from build123d import *

# Parameters (mm, degrees)
BOX_W             = 0.2
BOX_H             = 2.5
BOX_DEPTH         = 0.5
BOX001_W          = 2.5
BOX001_H          = 0.2
BOX001_DEPTH      = 0.5
CYLINDER_R        = 2.8
CYLINDER_DEPTH    = 1.65
CYLINDER001_R     = 1
CYLINDER001_DEPTH = 5
CHAMFER_SIZE      = 1.59
CHAMFER001_SIZE   = 0.1


with BuildPart() as obj1:
    # Box → Box (new body)
    with BuildSketch(Plane(origin=(-0.1, -1.25, 0), x_dir=(1, 0, 0), z_dir=(0, 0, 1))):
        with Locations((0.1, 1.25)):
            Rectangle(BOX_W, BOX_H)
    extrude(amount=BOX_DEPTH)


with BuildPart() as fusion:
    # Box001 → Box001 (new body)
    with BuildSketch(Plane(origin=(-1.25, -0.1, 0), x_dir=(1, 0, 0), z_dir=(0, 0, 1))):
        with Locations((1.25, 0.1)):
            Rectangle(BOX001_W, BOX001_H)
    extrude(amount=BOX001_DEPTH)

    # Fusion: union obj1
    add(obj1.part)


with BuildPart() as zylinder:
    # Cylinder → Cylinder (new body)
    with BuildSketch(Plane.XY):
        Circle(CYLINDER_R)
    extrude(amount=CYLINDER_DEPTH)


with BuildPart() as screw:
    # Cylinder001 → Cylinder001 (new body)
    with BuildSketch(Plane.XY.offset(0.1)):
        Circle(CYLINDER001_R)
    extrude(amount=CYLINDER001_DEPTH)

    # Fusion001: union Zylinder
    add(zylinder.part)

    # Cut: cut Fusion
    add(fusion.part, mode=Mode.SUBTRACT)

    # Chamfer
    chamfer_edges = [screw.edges().sort_by_distance(p)[0] for p in [
        (-2.8, 0, 1.65),
    ]]
    chamfer(chamfer_edges, length=CHAMFER_SIZE)

    # Chamfer001
    chamfer001_edges = [screw.edges().sort_by_distance(p)[0] for p in [
        (-1, 0, 5.1),
    ]]
    chamfer(chamfer001_edges, length=CHAMFER001_SIZE)


solid = screw.part
Can you work these out from the model? Positions are in its coordinate system, mm. Round coordinates to 2 decimals unless told otherwise and drop trailing zeros. Write each loop counter-clockwise with the first axis right and the second up, starting at its lowest first coordinate (ties: lowest second). Pieces come first, ordered by that corner, then holes. Notation, with made-up numbers: M 33,42 L 61,42 A17 ccw 61,59 Z; hole C 66,-13 d8. An arc over 180 degrees is marked long. Use a Markdown table: item, result.
Item 1: I want a section at C-C (z = 3.9). List the corners of the cut face in (x, y) for me.
Found:
| item | result |
|---|---|
| outline | C 0,0 d2 |
Item 2: For pin 1 Ø2 at (x, y) = (-0.5, 1) entering from +Z; pin 2 Ø1.5 at (x, y) = (2, 1.5) entering from +Z; pin 3 Ø0.6 at (y, z) = (1, 0.5) entering from +X; pin 4 Ø2 at (x, z) = (-1, 2.5) entering from -Y, each with a flat end and sliding along its axis, tell me the tip position at first contact or that it passes through.
Found:
| item | result |
|---|---|
| pin 1 | stops at z = 5.1 |
| pin 2 | stops at z = 1.11 |
| pin 3 | stops at x = 2.48 |
| pin 4 | stops at y = -1.13 |
Item 3: We'd pull the mould along Y, two halves only. Please class faces 1 (the face through (0, -1, 3)), 2 (the face through (0, 0, 5.1)): released by +Y, released by -Y, zero draft, split by the parting line, or undercut.
Found:
| item | result |
|---|---|
| face 1 | split by the parting line |
| face 2 | zero draft |
Item 4: If I drill on line 1 along X through (y, z) = (0, 4.7); line 2 along X through (y, z) = (-1.65, 1); line 3 along Y through (x, z) = (0.45, 2.2), over which ranges is the centre line in solid material (lowest first)? Write a range as [from, to].
Found:
| item | result |
|---|---|
| line 1 | x = [-1, 1] |
| line 2 | x = [-0.86, 0.86] |
| line 3 | y = [-0.89, 0.89] |
Item 5: I want a section at A-A (x = 0). List the corners of the cut face in (y, z) for me, and give its area (3 significant figures).
Found:
| item | result |
|---|---|
| outline | M -2.8,0 L -1.25,0 L -1.25,0.5 L 1.25,0.5 L 1.25,0 L 2.8,0 L 2.8,0.06 L 1.21,1.65 L 1,1.65 L 1,5 L 0.9,5.1 L -0.9,5.1 L -1,5 L -1,1.65 L -1.21,1.65 L -2.8,0.06 Z |
| area | 12.4 mm2 |
